```python
from build123d import *

# Parameters (mm, degrees)
TABAN_FLAN_1_DEPTH          = 5
IZIM8_R                     = 4.25
KES_EKSTR_ZYON1_DEPTH       = 10
RADYUS1_R                   = 20
RADYUS2_R                   = 5
RADYUS3_R                   = 2
IZIM10_W                    = 5
IZIM10_H                    = 20
Y_KSEKLIK_EKSTR_ZYON1_DEPTH = 4


# Sheet-metal steps are written as plain solids
with BuildPart() as part:
    # Çizim1 → Taban-Flanş1 (new body)
    with BuildSketch(Plane.XY):
        Polygon((0, 0), (-45, 0), (-85, -60), (-85, -115), (-15, -115), (-15, -60), (0, -60), align=None)
    extrude(amount=-TABAN_FLAN_1_DEPTH)

    # Çizim8 → Kes-Ekstrüzyon1 (cut)
    with BuildSketch(Plane.XY):
        with Locations((-35, -90)):
            Circle(IZIM8_R)
        with Locations((-60, -90)):
            Circle(IZIM8_R)
    extrude(amount=-KES_EKSTR_ZYON1_DEPTH, mode=Mode.SUBTRACT)

    # Radyus1
    radyus1_edges = [part.edges().sort_by_distance(p)[0] for p in [
        (-85, -60, -2.5),
        (-45, 0, -2.5),
    ]]
    fillet(radyus1_edges, radius=RADYUS1_R)

    # Radyus2
    radyus2_edges = [part.edges().sort_by_distance(p)[0] for p in [
        (-15, -60, -2.5),
        (-15, -115, -2.5),
        (-85, -115, -2.5),
    ]]
    fillet(radyus2_edges, radius=RADYUS2_R)

    # Radyus3
    radyus3_edges = [part.edges().sort_by_distance(p)[0] for p in [
        (0, -60, -2.5),
        (0, 0, -2.5),
    ]]
    fillet(radyus3_edges, radius=RADYUS3_R)

    # Çizim10 → Yükseklik-Ekstrüzyon1 (add)
    with BuildSketch(Plane(origin=(0, 0, 0), x_dir=(0, 0, -1), z_dir=(1, 0, 0))):
        with Locations((2.5, -30)):
            Rectangle(IZIM10_W, IZIM10_H)
    extrude(amount=Y_KSEKLIK_EKSTR_ZYON1_DEPTH)


solid = part.part
```
For this review, take the finished solid that the model builds, in its own axes (mm). A direction names the side the tool comes from. Coordinates: 2 decimals unless noted, no trailing zeros. Loops run counter-clockwise (first coordinate to the right, second up) from the corner with the lowest first, then second, coordinate; pieces in that order, holes last. Notation, with made-up numbers: (10, 45) - (30, 45) arc R20 cw to (30, 71) - close; hole circle Ø5 at (-34, 62.25). An arc over 180 degrees is marked (long way). Use one line per item in the form item = value. Start each with the question number.
1) For pin 1 (2.5 mm diameter, centred on y = -10.5, z = -3, fed in from +X); pin 2 (2 mm diameter, centred on x = 2, z = -2.5, fed in from -Y), all flat-tipped, find the tip position at first contact; note any pin that passes through.
2) Draft analysis for pull direction Y (two halves, no side actions). For faces 1 (the face through (-38.37, -92.59, -2.46)), 2 (the face through (-66.074, -31.611, -2.465)), 3 (the face through (2, -40, -2)), state which applies: released by +Y, released by -Y, zero draft, split by the parting line, or undercut.
3) Take a section at A-A (y = -90). State the section outline as (x, z) points, plus the area to 3 significant figures.
4) Take a section at C-C (z = -2.25). State the section outline as (x, y) points, plus the area to 3 significant figures.
5) Take a section at B-B (x = -60). State the section outline as (y, z) points.
6) To check wall thickness, follow probe 1 along Y at (x, z) = (-35, -2.4); probe 2 along X at (y, z) = (-72, -0.85); probe 3 along Y at (x, z) = (-61.5, -0.45). State the ranges of each line that lie inside material, in increasing order. Write a range as from..to.
7) For faces 4 (the face through (-41, -57, -5)), 5 (the face through (-15, -88, -2)), 6 (the face through (2, -20, -2)), list the 3-axis set-ups (+Z, -Z, +X, -X, +Y, -Y) from which the entire face can be reached by the end or side of a thin tool; tool diameter is ignored.
8) Take a section at D-D (y = -12). State the section outline as (x, z) points.
From the geometry:
q1.pin_1 = 0
q1.pin_2 = -40
q2.face_1 = undercut
q2.face_2 = released by +Y
q2.face_3 = released by -Y
q3.outline = (-85, -5) - (-64.25, -5) - (-64.25, 0) - (-85, 0) - close; (-55.75, -5) - (-39.25, -5) - (-39.25, 0) - (-55.75, 0) - close; (-30.75, -5) - (-15, -5) - (-15, 0) - (-30.75, 0) - close
q3.area = 265 mm2
q4.outline = (-85, -110) arc R5 ccw to (-80, -115) - (-20, -115) arc R5 ccw to (-15, -110) - (-15, -65) arc R5 cw to (-10, -60) - (-2, -60) arc R2 ccw to (0, -58) - (0, -40) - (4, -40) - (4, -20) - (0, -20) - (0, -2) arc R2 ccw to (-2, 0) - (-34.3, 0) arc R20 ccw to (-50.94, -8.91) - (-81.64, -54.96) arc R20 ccw to (-85, -66.06) - close; hole circle Ø8.5 at (-60, -90); hole circle Ø8.5 at (-35, -90)
q4.area = 7,690 mm2
q5.outline = (-115, -5) - (-94.25, -5) - (-94.25, 0) - (-115, 0) - close; (-85.75, -5) - (-22.5, -5) - (-22.5, 0) - (-85.75, 0) - close
q6.probe_1 = -115..-94.25, -85.75..-0.01
q6.probe_2 = -85..-15
q6.probe_3 = -115..-93.98, -86.02..-24.75
q7.face_4 = -Z, +X, -X, +Y, -Y
q7.face_5 = +Z, -Z, +X, -Y
q7.face_6 = +Z, -Z, +X, +Y
q8.outline = (-53, -5) - (0, -5) - (0, 0) - (-53, 0) - close
